Input: part model. Units: mm. Frame: model coordinates. A direction names the side the tool comes from. Coordinates: 2 decimals unless noted, no trailing zeros. Order: outer loops, then holes, each group sorted by start corner. A loop starts at its lowest first (then second) coordinate and runs counter-clockwise, first axis right, second up. Notation, with made-up numbers: M 59.5,63.25 L 65.5,63.25 A34 cw 65.5,100.25 Z; hole C 13,45.5 d3. An arc over 180 degrees is marked long. One line per item, written item: value.
```python
from build123d import *

# Parameters (mm, degrees)
SKETCH1_W                      = 593
SKETCH1_H                      = 660.6
BASE_FLANGE1_DEPTH             = 2.7
EDGE_FLANGE1_STRIP_W           = 14.8
EDGE_FLANGE1_STRIP_H           = 2.7
EDGE_FLANGE1_STRIP_CUT_DEPTH   = 660.6
EDGE_FLANGE1_STRIP_2_W         = 14.8
EDGE_FLANGE1_STRIP_2_H         = 2.7
EDGE_FLANGE1_STRIP_CUT_2_DEPTH = 660.6
EDGE_FLANGE1_DEPTH             = 660.6
EDGE_FLANGE1_BEND_DEPTH        = 660.6
EDGE_FLANGE2_STRIP_W           = 14.8
EDGE_FLANGE2_STRIP_H           = 2.7
EDGE_FLANGE2_STRIP_CUT_DEPTH   = 583.6
EDGE_FLANGE2_DEPTH             = 583.6
CUT_EXTRUDE2_REACH             = 891.9
SKETCH15_W                     = 38.6
SKETCH15_H                     = 5.3
SKETCH15_W_2                   = 55
EDGE_FLANGE3_STRIP_W           = 14.8
EDGE_FLANGE3_STRIP_H           = 2.7
EDGE_FLANGE3_STRIP_CUT_DEPTH   = 583.6
EDGE_FLANGE3_DEPTH             = 583.6
CUT_EXTRUDE3_REACH             = 891.9
SKETCH23_W                     = 170
SKETCH23_H                     = 5


# Sheet-metal steps are written as plain solids
with BuildPart() as part:
    # Sketch1 → Base-Flange1 (new body)
    with BuildSketch(Plane.XY):
        with Locations((296.5, 330.3)):
            Rectangle(SKETCH1_W, SKETCH1_H)
    extrude(amount=-BASE_FLANGE1_DEPTH)

    # Edge-Flange1 strip (across the edge) → Edge-Flange1 strip cut (cut)
    with BuildSketch(Plane.XZ.offset(-660.6)):
        with Locations((-2.7, -1.35)):
            Rectangle(EDGE_FLANGE1_STRIP_W, EDGE_FLANGE1_STRIP_H)
    extrude(amount=EDGE_FLANGE1_STRIP_CUT_DEPTH, mode=Mode.SUBTRACT)

    # Edge-Flange1 strip 2 (across the edge) → Edge-Flange1 strip cut 2 (cut)
    with BuildSketch(Plane(origin=(593, 0, 0), x_dir=(-1, 0, 0), z_dir=(0, 1, 0))):
        with Locations((-2.7, -1.35)):
            Rectangle(EDGE_FLANGE1_STRIP_2_W, EDGE_FLANGE1_STRIP_2_H)
    extrude(amount=EDGE_FLANGE1_STRIP_CUT_2_DEPTH, mode=Mode.SUBTRACT)

    # Edge-Flange1 section (across the edge) → Edge-Flange1 (add)
    with BuildSketch(Plane.XZ.offset(-660.6)):
        with BuildLine():
            Line((0, 2), (0, 62.3))
            Line((0, 62.3), (2.7, 62.3))
            Line((2.7, 62.3), (2.7, 2))
            ThreePointArc((2.7, 2), (3.285786438, 0.585786438), (4.7, 0))
            Line((4.7, 0), (4.7, -2.7))
            ThreePointArc((4.7, -2.7), (1.376598128, -1.323401872), (0, 2))
        make_face()
    extrude(amount=EDGE_FLANGE1_DEPTH)

    # Edge-Flange1 section 2 (across the edge) → Edge-Flange1 bend (add)
    with BuildSketch(Plane(origin=(593, 0, 0), x_dir=(-1, 0, 0), z_dir=(0, 1, 0))):
        with BuildLine():
            Line((0, 2), (0, 62.3))
            Line((0, 62.3), (2.7, 62.3))
            Line((2.7, 62.3), (2.7, 2))
            ThreePointArc((2.7, 2), (3.285786438, 0.585786438), (4.7, 0))
            Line((4.7, 0), (4.7, -2.7))
            ThreePointArc((4.7, -2.7), (1.376598128, -1.323401872), (0, 2))
        make_face()
    extrude(amount=EDGE_FLANGE1_BEND_DEPTH)

    # Edge-Flange2 strip (across the edge) → Edge-Flange2 strip cut (cut)
    with BuildSketch(Plane(origin=(588.3, 660.6, 0), x_dir=(0, -1, 0), z_dir=(-1, 0, 0))):
        with Locations((-2.7, -1.35)):
            Rectangle(EDGE_FLANGE2_STRIP_W, EDGE_FLANGE2_STRIP_H)
    extrude(amount=EDGE_FLANGE2_STRIP_CUT_DEPTH, mode=Mode.SUBTRACT)

    # Edge-Flange2 section (across the edge) → Edge-Flange2 (add)
    with BuildSketch(Plane(origin=(588.3, 660.6, 0), x_dir=(0, -1, 0), z_dir=(-1, 0, 0))):
        with BuildLine():
            Line((0, 2), (0, 7.3))
            Line((0, 7.3), (2.7, 7.3))
            Line((2.7, 7.3), (2.7, 2))
            ThreePointArc((2.7, 2), (3.285786438, 0.585786438), (4.7, 0))
            Line((4.7, 0), (4.7, -2.7))
            ThreePointArc((4.7, -2.7), (1.376598128, -1.323401872), (0, 2))
        make_face()
    extrude(amount=EDGE_FLANGE2_DEPTH)

    # Sketch15 → Cut-Extrude2 (cut, up to next)
    with BuildSketch(Plane(origin=(0, 660.6, 0), x_dir=(1, 0, 0), z_dir=(0, 1, 0)), mode=Mode.PRIVATE) as cut_extrude2_sk1:
        with Locations((24, -4.65)):
            Rectangle(SKETCH15_W, SKETCH15_H)
    cut_extrude2_tool1 = extrude(cut_extrude2_sk1.sketch, amount=-CUT_EXTRUDE2_REACH, mode=Mode.PRIVATE) & part.part
    # Sketch15 → Cut-Extrude2 (cut, up to next)
    with BuildSketch(Plane(origin=(0, 660.6, 0), x_dir=(1, 0, 0), z_dir=(0, 1, 0)), mode=Mode.PRIVATE) as cut_extrude2_sk2:
        with Locations((210.8, -4.65)):
            Rectangle(SKETCH15_W_2, SKETCH15_H)
    cut_extrude2_tool2 = extrude(cut_extrude2_sk2.sketch, amount=-CUT_EXTRUDE2_REACH, mode=Mode.PRIVATE) & part.part
    # Sketch15 → Cut-Extrude2 (cut, up to next)
    with BuildSketch(Plane(origin=(0, 660.6, 0), x_dir=(1, 0, 0), z_dir=(0, 1, 0)), mode=Mode.PRIVATE) as cut_extrude2_sk3:
        with Locations((365.8, -4.65)):
            Rectangle(SKETCH15_W_2, SKETCH15_H)
    cut_extrude2_tool3 = extrude(cut_extrude2_sk3.sketch, amount=-CUT_EXTRUDE2_REACH, mode=Mode.PRIVATE) & part.part
    # Sketch15 → Cut-Extrude2 (cut, up to next)
    with BuildSketch(Plane(origin=(0, 660.6, 0), x_dir=(1, 0, 0), z_dir=(0, 1, 0)), mode=Mode.PRIVATE) as cut_extrude2_sk4:
        with Locations((560.8, -4.65)):
            Rectangle(SKETCH15_W_2, SKETCH15_H)
    cut_extrude2_tool4 = extrude(cut_extrude2_sk4.sketch, amount=-CUT_EXTRUDE2_REACH, mode=Mode.PRIVATE) & part.part
    add(cut_extrude2_tool1.solids().sort_by_distance((24, 660.6, 4.65))[0], mode=Mode.SUBTRACT)
    add(cut_extrude2_tool2.solids().sort_by_distance((210.8, 660.6, 4.65))[0], mode=Mode.SUBTRACT)
    add(cut_extrude2_tool3.solids().sort_by_distance((365.8, 660.6, 4.65))[0], mode=Mode.SUBTRACT)
    add(cut_extrude2_tool4.solids().sort_by_distance((560.8, 660.6, 4.65))[0], mode=Mode.SUBTRACT)

    # Edge-Flange3 strip (across the edge) → Edge-Flange3 strip cut (cut)
    with BuildSketch(Plane.YZ.offset(4.7)):
        with Locations((-2.7, -1.35)):
            Rectangle(EDGE_FLANGE3_STRIP_W, EDGE_FLANGE3_STRIP_H)
    extrude(amount=EDGE_FLANGE3_STRIP_CUT_DEPTH, mode=Mode.SUBTRACT)

    # Edge-Flange3 section (across the edge) → Edge-Flange3 (add)
    with BuildSketch(Plane.YZ.offset(4.7)):
        with BuildLine():
            Line((0, 2), (0, 17.3))
            Line((0, 17.3), (2.7, 17.3))
            Line((2.7, 17.3), (2.7, 2))
            ThreePointArc((2.7, 2), (3.285786438, 0.585786438), (4.7, 0))
            Line((4.7, 0), (4.7, -2.7))
            ThreePointArc((4.7, -2.7), (1.376598128, -1.323401872), (0, 2))
        make_face()
    extrude(amount=EDGE_FLANGE3_DEPTH)

    # Sketch23 → Cut-Extrude3 (cut, up to next)
    with BuildSketch(Plane.XZ, mode=Mode.PRIVATE) as cut_extrude3_sk1:
        with Locations((296.5, 14.8)):
            Rectangle(SKETCH23_W, SKETCH23_H)
    cut_extrude3_tool1 = extrude(cut_extrude3_sk1.sketch, amount=-CUT_EXTRUDE3_REACH, mode=Mode.PRIVATE) & part.part
    add(cut_extrude3_tool1.solids().sort_by_distance((296.5, 0, 14.8))[0], mode=Mode.SUBTRACT)


solid = part.part
```
(1) Access query for faces 1 (the flat face through (593, 326, 32)), 2 (the flat face through (2.7, 335, 33)). Directions: +Z, -Z, +X, -X, +Y, -Y. A direction counts if a zero-diameter tool reaches every point of the face in a straight line with its end or side. Return the directions, or none.
Data:
face 1: +Z, -Z, +X, +Y, -Y
face 2: +Z, +Y, -Y
(2) Cut plane D-D on x = 57. Output: boundary loops of the cut face in (y, z), plus the area to 3 significant figures.
Data:
outline: M 0,2 A4.7 ccw 4.7,-2.7 L 655.9,-2.7 A4.7 ccw 660.6,2 L 660.6,7.3 L 657.9,7.3 L 657.9,2 A2 cw 655.9,0 L 4.7,0 A2 cw 2.7,2 L 2.7,17.3 L 0,17.3 Z
area: 1,840 mm2
(3) Cut plane C-C on y = 362.5. Output: boundary loops of the cut face in (x, z), plus the area to 3 significant figures.
Data:
outline: M 0,2 A4.7 ccw 4.7,-2.7 L 588.3,-2.7 A4.7 ccw 593,2 L 593,62.3 L 590.3,62.3 L 590.3,2 A2 cw 588.3,0 L 4.7,0 A2 cw 2.7,2 L 2.7,62.3 L 0,62.3 Z
area: 1,930 mm2
(4) First-contact query: pin 1 (10 mm diameter, centred on x = 76, z = 24, fed in from +Y); pin 2 (3 mm diameter, centred on x = 256, y = 1.5, fed in from +Z); pin 3 (2 mm diameter, centred on x = 569, y = 660, fed in from +Z); pin 4 (2 mm diameter, centred on x = 463.5, y = 659.5, fed in from +Z). Flat tips, straight axial feed; report the tip coordinate or a pass-through.
Data:
pin 1: passes through
pin 2: stops at z = 12.3
pin 3: stops at z = 2
pin 4: stops at z = 7.3
(5) Draft query along Y for faces 3 (the flat face through (292, 335, 0)), 4 (the flat face through (590.3, 326, 33)), 5 (the flat face through (292, 2.7, 10)), 6 (the flat face through (292, 0, 10)). Return one class per face: released by +Y, released by -Y, zero draft, split by the parting line, or undercut.
Data:
face 3: undercut
face 4: zero draft
face 5: undercut
face 6: released by -Y
(6) Ray query, line 1 (X direction, y = 377, z = 30.5); line 2 (Y direction, x = 453.5, z = 3); line 3 (Y direction, x = 140.5, z = 14.5). Return the intervals inside material, ascending. Write a range as from..to.
Data:
line 1: x = 0..2.7, 590.3..593
line 2: y = 0..2.7, 657.9..660.6
line 3: y = 0..2.7
(7) Cut plane A-A on z = 49. Output: boundary loops of the cut face in (x, y), plus the area to 3 significant figures.
Data:
outline: M 0,0 L 2.7,0 L 2.7,660.6 L 0,660.6 Z; M 590.3,0 L 593,0 L 593,660.6 L 590.3,660.6 Z
area: 3,570 mm2
(8) Cut plane B-B on x = 362. Output: boundary loops of the cut face in (y, z).
Data:
outline: M 0,2 A4.7 ccw 4.7,-2.7 L 655.9,-2.7 A4.7 ccw 660.6,2 L 657.9,2 A2 cw 655.9,0 L 4.7,0 A2 cw 2.7,2 L 2.7,12.3 L 0,12.3 Z
